from build123d import *

# Parameters (mm, degrees)
F1_ANGLE = 90
F2_R     = 5.08


with BuildPart() as f1:
    # F0 (on Front) → F1 (revolve)
    with BuildSketch(Plane.XZ):
        Polygon((45.896156, 50.8), (5.719585, 50.8), (5.719585, 28.575), (68.21648, 28.575), (68.21648, 38.1), (45.896156, 38.1), align=None)
    revolve(axis=Axis((39.269814, 0, 0), (1, 0, 0)), revolution_arc=F1_ANGLE)

    # F2
    f2_edges = [f1.edges().sort_by_distance(p)[0] for p in [
        (45.896156, -26.940768, 26.940768),
    ]]
    fillet(f2_edges, radius=F2_R)


solid = f1.part
Work out the finished part from the listing and answer in its coordinate system (mm). A direction names the side the tool comes from. Give positions to 0.01 mm unless a question says otherwise; leave off trailing zeros. Order: outer loops, then holes, each group sorted by start corner. A loop starts at its lowest first (then second) coordinate and runs counter-clockwise, first axis right, second up. Notation, with made-up numbers: (-3, 41) - (36, 41) arc R38 ccw to (36, 80) - close; hole circle Ø8 at (51.5, 76.5). An arc over 180 degrees is marked (long way). Answer as CSV lines item,"result". Start each with the question number.
Q1. Find the intervals of material crossed by L1, parallel to X at y = -46, z = 7; L2, parallel to X at y = -10, z = 38.5; L3, parallel to Z at x = 39, y = -20, in increasing order. Write a range as [from, to].
Q2. The part is cut by section A-A (x = 60). Write down the section's boundary in (y, z) (3 decimals), then the cut area to 3 significant figures.
Q3. For faces 1 (the face through (59.48, -26.64, 27.24)), 2 (the face through (5.72, -26, 25)), determine the directions among +Z, -Z, +X, -X, +Y, -Y from which every point of the face is accessible in a straight line to the end or side of a thin tool.
Q4. Given pin 1 Ø6 at (x, z) = (53.5, 16.5) entering from -Y; pin 2 Ø4 at (x, z) = (40, 26.5) entering from -Y; pin 3 Ø1.5 at (x, y) = (26.5, -24.5) entering from -Z, each flat-ended and moving along its own axis, determine where each tip first touches the part or whether it passes through.
Q5. The part is cut by section B-B (z = 46). Write down the section's boundary in (x, y), then the cut area to 3 significant figures.
Check result:
1,L1,"x = [5.72, 45.9]"
1,L2,"x = [5.72, 47.2]"
1,L3,"z = [20.41, 46.7]"
2,outline,"(-38.1, 0) - (-28.575, 0) arc R28.575 cw to (0, 28.575) - (0, 38.1) arc R38.1 ccw to start"
2,area,"499 mm²"
3,face 1,"+Z, +X, -Y"
3,face 2,"+Z, -Z, -X, +Y, -Y"
4,pin 1,"stops at y = -35.63"
4,pin 2,"stops at y = -44.5"
4,pin 3,"stops at z = 13.38"
5,outline,"(5.72, -21.56) - (45.9, -21.56) - (45.9, 0) - (5.72, 0) - close"
5,area,"866 mm²"
